Design review of the part built by this model. Coordinates are the model's own, in mm. Give positions to 0.01 mm unless a question says otherwise; leave off trailing zeros. Order: outer loops, then holes, each group sorted by start corner. A loop starts at its lowest first (then second) coordinate and runs counter-clockwise, first axis right, second up. Notation, with made-up numbers: (33, 0) -> (75, 0) arc R21 cw to (75, 31) -> close; hole circle Ø2 at (58, 11.25). An arc over 180 degrees is marked (long way). Answer in a Markdown table with one row per item. Add a question column.
```python
from build123d import *

# Parameters (mm, degrees)
BOSS_EXTRUDE1_DEPTH = 40
FILLET1_R           = 0.5


with BuildPart() as part:
    # Sketch1 → Boss-Extrude1 (new body)
    with BuildSketch(Plane(origin=(0, 0, 0), x_dir=(-1, 0, 0), z_dir=(0, 1, 0))):
        Polygon((7.745479892, -18.700646836), (-7.74610734, -18.700646836), (-18.700313724, -7.746440452), (-18.700313724, 7.745146781), (-7.74610734, 18.699353164), (7.745479892, 18.699353164), (18.699686276, 7.745146781), (18.699686276, -7.746440452), align=None)
    extrude(amount=BOSS_EXTRUDE1_DEPTH)

    # Fillet1
    fillet1_edges = [part.edges().sort_by_distance(p)[0] for p in [
        (0.000313724, 0, 18.699353164),
        (-13.222583084, 0, 13.222249973),
        (-18.699686276, 0, -0.000646836),
        (-13.222583084, 0, -13.223543644),
        (-13.222583084, 40, 13.222249973),
        (0.000313724, 40, 18.699353164),
        (13.223210532, 40, 13.222249973),
        (18.700313724, 40, -0.000646836),
        (13.223210532, 40, -13.223543644),
        (0.000313724, 40, -18.700646836),
        (-13.222583084, 40, -13.223543644),
        (0.000313724, 0, -18.700646836),
        (-18.699686276, 40, -0.000646836),
        (13.223210532, 0, -13.223543644),
        (18.700313724, 0, -0.000646836),
        (13.223210532, 0, 13.222249973),
    ]]
    fillet(fillet1_edges, radius=FILLET1_R)


solid = part.part
```
1) Add section A-A, the plane y = 13. Write out the cut boundary in (x, z), and give its area (3 significant figures).
2) Clearance check with flat-ended pins moving along their axes: P1, Ø5, axis at y = 33.5, z = -12.5, coming from the -X side; P2, Ø12, axis at x = -14.5, y = 7, coming from the -Z side; P3, Ø5, axis at y = 10.5, z = 12, coming from the -X side. State where each tip first meets the part, or that it passes through.
3) For L1, parallel to X at y = 10, z = 17.5; L2, parallel to X at y = 30, z = -16.5; L3, parallel to Z at x = -13, y = 9, list the stretches that pass through material, from the lowest coordinate up.
Verdict:
| question | item | result |
|---|---|---|
| 1 | outline | (-18.7, -7.75) -> (-7.75, -18.7) -> (7.75, -18.7) -> (18.7, -7.75) -> (18.7, 7.75) -> (7.75, 18.7) -> (-7.75, 18.7) -> (-18.7, 7.75) -> close |
| 1 | area | 1,160 mm2 |
| 2 | P1 | stops at x = -16.45 |
| 2 | P2 | stops at z = -17.95 |
| 2 | P3 | stops at x = -16.94 |
| 3 | L1 | x = -8.94 to 8.95 |
| 3 | L2 | x = -9.95 to 9.95 |
| 3 | L3 | z = -13.45 to 13.44 |
